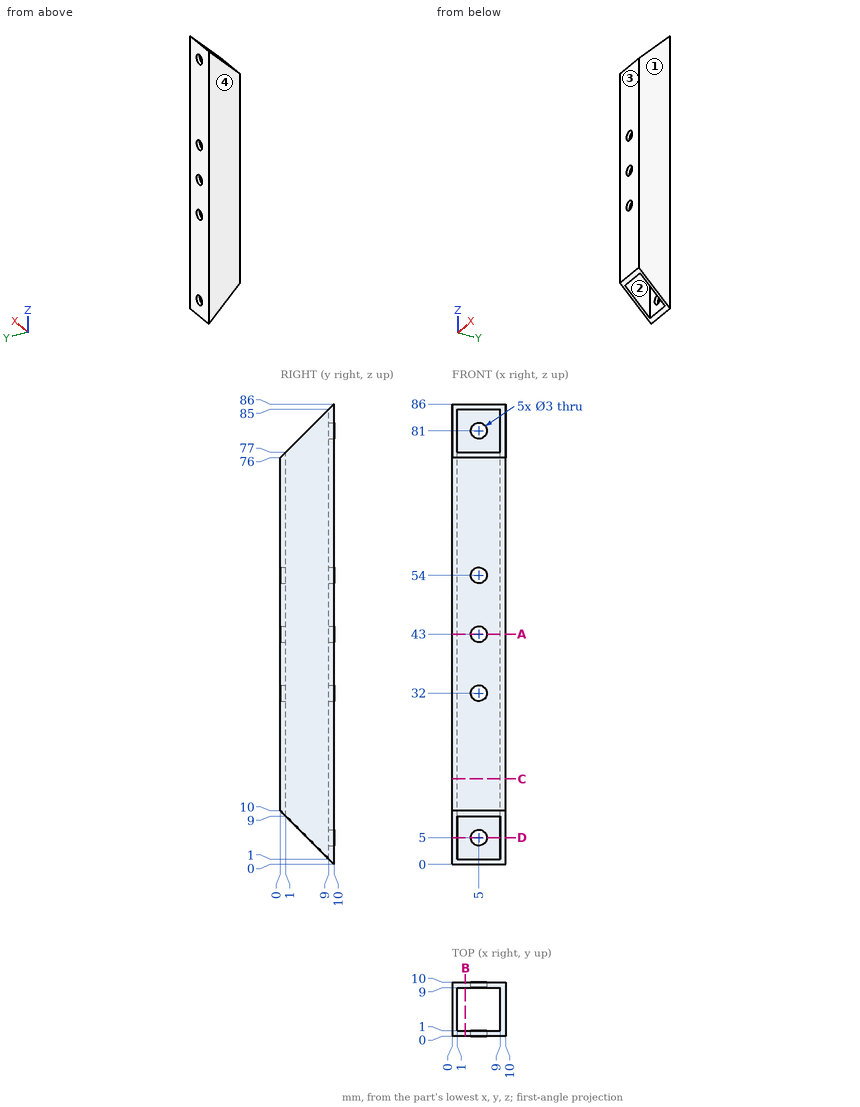
Verification items for this drawing (mm, ordinates from the low corner). Give positions to 0.01 mm unless a question says otherwise; leave off trailing zeros. Loops run counter-clockwise (first coordinate to the right, second up) from the corner with the lowest first, then second, coordinate; pieces in that order, holes last. Notation, with made-up numbers: M 89.5,-6 L 119.5,-6 A18 ccw 119.5,23 Z; hole C 62,1.5 d11. An arc over 180 degrees is marked long. Answer as a JSON object with one key per item and string values. Group by question number.
Item 1: Mould release check, pull along X, two halves, no side actions. Record for the marked faces 1, 2, 3 and 4: pulls with the +X half, pulls with the -X half, needs draft (parallel to the pull), parting line crosses it, or undercut.
Item 2: Gauge pin test, flat ends, axial feed: pin 1 (4 mm diameter, centred on x = 5, z = 81, fed in from -Y); pin 2 (1.8 mm diameter, centred on x = 5, z = 43, fed in from +Y); pin 3 (3 mm diameter, centred on x = 9, y = 7, fed in from +Z). Record the tip position at first contact, or that the pin passes through.
Item 3: Material ranges on L1, parallel to X at y = 0.4, z = 43; L2, parallel to Y at x = 5.75, z = 12, recorded low to high.
Item 4: Sectioned sample at C-C on z = 16. Record the boundary of the cut face in (x, y), plus the area to 3 significant figures.
Item 5: Sectioned sample at B-B on x = 2.5. Record the boundary of the cut face in (y, z).
Item 6: Sectioned sample at D-D on z = 5. Record the boundary of the cut face in (x, y).
Item 7: Sectioned sample at A-A on z = 43. Record the boundary of the cut face in (x, y).
Findings below:
{
 "1": {"face 1": "pulls with the +X half", "face 2": "undercut", "face 3": "needs draft", "face 4": "pulls with the -X half"},
 "2": {"pin 1": "y = 9", "pin 2": "through", "pin 3": "z = 84.5"},
 "3": {"L1": "0 to 3.5, 6.5 to 10", "L2": "0 to 1, 9 to 10"},
 "4": {"outline": "M 0,0 L 10,0 L 10,10 L 0,10 Z; hole M 1,1 L 9,1 L 9,9 L 1,9 Z", "area": "36.0 mm2"},
 "5": {"outline": "M 0,10 L 1,9 L 1,77 L 0,76 Z; M 9,1 L 10,0 L 10,86 L 9,85 Z"},
 "6": {"outline": "M 0,5 L 1,5 L 1,9 L 3.5,9 L 3.5,10 L 0,10 Z; M 6.5,9 L 9,9 L 9,5 L 10,5 L 10,10 L 6.5,10 Z"},
 "7": {"outline": "M 0,0 L 3.5,0 L 3.5,1 L 1,1 L 1,9 L 3.5,9 L 3.5,10 L 0,10 Z; M 6.5,0 L 10,0 L 10,10 L 6.5,10 L 6.5,9 L 9,9 L 9,1 L 6.5,1 Z"}
}
